Read the model definition and answer for the solid it produces. Units are mm, in the model's axes. A direction names the side the tool comes from. Give positions to 0.01 mm unless a question says otherwise; leave off trailing zeros. Loops run counter-clockwise (first coordinate to the right, second up) from the corner with the lowest first, then second, coordinate; pieces in that order, holes last. Notation, with made-up numbers: (51, 72.5) - (55, 72.5) arc R26 cw to (55, 87.5) - close; hole circle Ø7 at (33, -2). An arc over 180 degrees is marked (long way). Write item = value, one per line.
Autodesk Fusion 360 part; units mm, degrees
sketch "Sketch1" plane through (0, 0, 0) normal (0, 0, 1) x (1, 0, 0)
  line L0 (0, 0) -> (0, -4.5)
  line L1 (-16, -9) -> (18, -9) construction
  line L2 (0, -4.5) -> (-4, -9)
  line L3 (-4, -9) -> (-4, -30)
  line L4 (0, 0) -> (-3, 0)
  line L5 (-3, 0) -> (-3, -2.7268)
  line L6 (-4, -30) -> (-8, -30)
  line L7 (-8, -30) -> (-8, -10.933)
  line L8 (-3.5201, -4.0721) -> (-6.6997, -7.5697)
  arc A0 (-3.5201, -4.0721) -> (-3, -2.7268) centre (-5, -2.7268) ccw
  arc A1 (-6.6997, -7.5697) -> (-8, -10.933) centre (-3, -10.933) ccw
  point P0 (-3, -3.5)
  dimension "d1" = 4.5
  dimension "d2" = 4.5
  dimension "d3" = 21
  dimension "d4" = 3
  dimension "d5" = 3.5
  dimension "d6" = 4
  dimension "d7" = 2
  dimension "d8" = 5
extrude "Extrude1" add sketch "Sketch1" along normal blind 32
sketch "Sketch2" plane through (-8, 0, 0) normal (-1, 0, 0) x (0, -1, 0)
  line L0 (10.933, 0) -> (30, 0)
  line L1 (30, 0) -> (30, 32)
  line L2 (30, 32) -> (10.933, 32)
  line L3 (10.933, 32) -> (10.933, 0)
  line L4 (30, 0) -> (15, 0)
  line L5 (15, 0) -> (15, 32)
  line L6 (15, 32) -> (30, 32)
  line L7 (30, 32) -> (30, 0)
  dimension "d11" = 15
extrude "Extrude2" add sketch "Sketch2" along normal blind 22 contours L0 L1 L2 L4 L5 L6 L7
extrude "Extrude3" cut 1 faces at (-30, -20, 21.3333) along direction (1, 0, 0) blind 2
extrude "Extrude4" add 1 faces at (-21.3333, -15, 10.6667) along direction (0, 1, 0) blind 4
extrude "Extrude5" cut 1 faces at (-21.3333, -11, 10.6667) along direction (0, -1, 0) blind 50
sketch "Sketch4" plane through (-8, 0, 0) normal (-1, 0, 0) x (0, -1, 0)
  line L0 (30, 0) -> (30, 32)
  line L1 (30, 32) -> (11, 32)
  line L2 (11, 32) -> (11, 0)
  line L3 (11, 0) -> (30, 0)
  line L4 (30, 32) -> (17, 32)
  line L5 (17, 32) -> (17, 5)
  line L6 (17, 5) -> (30, 5)
  line L7 (30, 5) -> (30, 32)
  dimension "d23" = 27
extrude "Extrude6" cut sketch "Sketch4" against normal blind 2 contours L0 L1 L4 L5 L6 L7
extrude "Extrude7" cut 1 faces at (-7.3333, -17, 23) along direction (0, 1, 0) blind 5
1) A cutting plane is placed at A-A on z = 25.5. Determine the outline of the cut face in (x, y), then the cut area to 3 significant figures.
Output:
outline = (-8, -12) - (-6, -12) - (-6, -30) - (-4, -30) - (-4, -9) - (0, -4.5) - (0, 0) - (-3, 0) - (-3, -2.73) arc R2 cw to (-3.52, -4.07) - (-6.7, -7.57) arc R5 ccw to (-8, -10.93) - close
area = 79.4 mm²
2) Each of these flat-tipped pins is pushed along its axis until it touches: P1, Ø1.5, axis at y = -4.5, z = 23, coming from the -X side; P2, Ø0.6, axis at x = -7, y = -21, coming from the +Z side; P3, Ø0.8, axis at y = -1.5, z = 15.5, coming from the -X side. Where does it stop, or does it pass through?
Output:
P1 = -4.59
P2 = 5
P3 = -3
3) A cutting plane is placed at B-B on y = -13.5. Determine the outline of the cut face in (x, z), then the cut area to 3 significant figures.
Output:
outline = (-8, 0) - (-4, 0) - (-4, 32) - (-6, 32) - (-6, 5) - (-8, 5) - close
area = 74.0 mm²
4) Find the intervals of material crossed by probe 1 along X at (y, z) = (-14.5, 23); probe 2 along Y at (x, z) = (-5.5, 4.5); probe 3 along Y at (x, z) = (-7, 19), in increasing order.
Output:
probe_1 = -6 to -4
probe_2 = -30 to -6.25
probe_3 = -12 to -7.93
5) A tool of negligible diameter and unlimited length cuts with its end or side. For faces 1 (the face through (-4, -19, 16)), 2 (the face through (-6, -21, 19)), 3 (the face through (-3, -1, 16)), from which of +Z, -Z, +X, -X, +Y, -Y can it reach the whole face along a straight path? Write none if from no direction.
Output:
face_1 = +Z, -Z, +X, -Y
face_2 = +Z, -X, -Y
face_3 = +Z, -Z, -X, +Y
